Read the model definition and answer for the solid it produces. Units are mm, in the model's axes. Face numbers are marked on the shaded views. A direction names the side the tool comes from. Give positions to 0.01 mm unless a question says otherwise; leave off trailing zeros.
Autodesk Fusion 360 part; units mm, degrees
sketch "Skizze1" plane through (0, 0, 0) normal (0, 1, 0) x (1, 0, 0)
  line L0 (0, 0) -> (15, 0)
  line L1 (15, 0) -> (15, 8)
  line L2 (15, 8) -> (0, 8)
  line L3 (0, 8) -> (0, 0)
  line L4 (0, 8) -> (39.7107, 20)
  line L5 (39.7107, 20) -> (40, 19.0428)
  line L6 (40, 19.0428) -> (3.457, 8)
  line L7 (40, 19.0428) -> (40, 8)
  line L8 (40, 8) -> (15, 8)
  dimension "d1" = 15
  dimension "d2" = 8
  dimension "d3" = 1
  dimension "d4" = 20
  dimension "d5" = 40
extrude "Extrusion1" add sketch "Skizze1" along normal mid plane 50
ref_plane "Arbeitsebene1" through (39.8554, 0, -19.5214) normal (0.9572, 0, -0.2893) x (-0.2893, 0, -0.9572)
sketch "Skizze2" plane through (41.9259, 0, -12.6694) normal (0.9572, 0, -0.2893) x (-0.2893, 0, -0.9572)
  line L0 (6.658, 12.5) -> (-8.342, 12.5)
  line L1 (-8.342, 12.5) -> (-8.342, -12.5)
  line L2 (-8.342, -12.5) -> (6.658, -12.5)
  line L3 (6.658, -12.5) -> (6.658, 12.5)
  line L4 (6.658, 12.5) -> (-8.342, -12.5) construction
  line L5 (-8.342, 12.5) -> (6.658, -12.5) construction
  line L6 (6.658, -25) -> (6.658, 25)
  point P0 (-0.842, 0)
  dimension "d11" = 15
  dimension "d23" = 25
extrude "Extrusion2" cut sketch "Skizze2" against normal blind 50
sketch "Skizze3" plane through (40, 0, 0) normal (1, 0, 0) x (0, 0, -1)
  line L0 (8, 12.5) -> (19.0428, 12.5)
  line L1 (19.0428, 12.5) -> (19.0428, 25)
  line L2 (19.0428, 25) -> (8, 25)
  line L3 (8, 25) -> (8, 12.5)
  line L4 (20, -25) -> (20, 25)
  line L5 (20, 25) -> (19.0428, 25)
  line L6 (19.0428, 25) -> (19.0428, 12.5)
  line L7 (19.0428, 12.5) -> (19.0428, -12.5)
  line L8 (19.0428, -12.5) -> (19.0428, -25)
  line L9 (19.0428, -25) -> (20, -25)
  line L10 (8, 12.5) -> (19.0428, 12.5)
  line L11 (19.0428, -12.5) -> (8, -12.5)
  line L12 (8, -12.5) -> (8, -25)
  line L13 (8, -25) -> (19.0428, -25)
  line L14 (19.0428, -25) -> (19.0428, -12.5)
  spline S0 degree 5 poles (20, -12.5) (20, -13.0888) (19.7652, -14.2211) (18.7091, -15.7836) (16.1706, -17.6488) (12.3294, -19.8512) (9.7909, -21.7164) (8.7348, -23.2789) (8.5, -24.4112) (8.5, -25) knots 0 0 0 0 0 0 0.2 0.4 0.6 0.8 1 1 1 1 1 1
  line L15 (20, -11.5) -> (20, -13.5)
  line L16 (8.5, -24) -> (8.5, -26)
  dimension "d14" = 2
  dimension "d15" = 2
  dimension "d16" = 0.5
extrude "Extrusion3" cut sketch "Skizze3" against normal blind 50 contours L4 L8 L9 L14 S0 L15 | L8 L13 L14 S0
extrude "Extrusion4" add 2 faces at (31.6667, -16.6667, -8) (31.6667, 16.6667, -8) along direction (0, 0, 1) blind 0.5
mirror "Spiegeln1" about plane through (0, 0, 0) normal (0, 1, 0) of "Extrusion3"
fillet "Abrundung1" radius 2 2 edges at (20, -12.5, -12.999) (20, 12.5, -12.999)
sketch "Skizze4" plane through (0, 12.5, 0) normal (0, -1, 0) x (1, 0, 0)
  line L0 (0, -4.866) -> (40, -16.9534)
  line L1 (40, -16.9534) -> (40, -7.5)
  line L2 (40, -7.5) -> (15, -7.5)
  line L3 (15, -7.5) -> (15, 0)
  line L4 (15, 0) -> (0, 0)
  line L5 (0, 0) -> (0, -4.866)
  line L6 (15, 0) -> (40, -7.5)
extrude "Extrusion5" add sketch "Skizze4" against normal blind 0.6 contours L2 L3 L6
mirror "Spiegeln2" about plane through (0, 0, 0) normal (0, 1, 0) of "Extrusion5"
equation "d15 = d14"
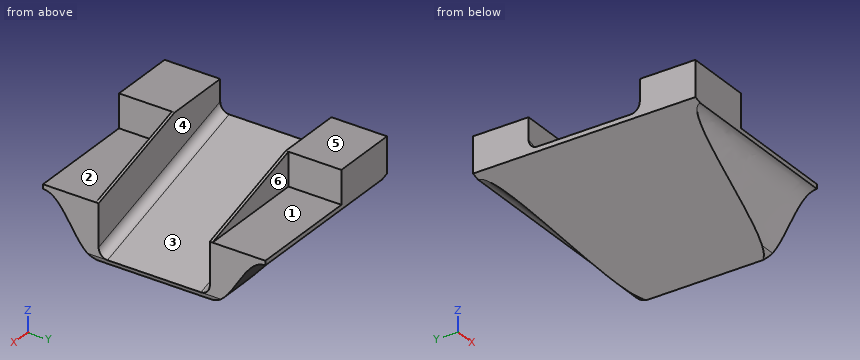
Item 1: Which of the six approach directions +Z, -Z, +X, -X, +Y, -Y give full straight-line access (tool end or side, diameter ignored) to the marked faces 1, 2 and 3?
Result set:
face 1: +Z, +X, +Y
face 2: +Z, +X, -Y
face 3: +Z, +X
Item 2: Find the intervals of material crossed by line 1 along Y through (x, z) = (23, -6); line 2 along Y through (x, z) = (2, -2); line 3 along X through (y, z) = (-13.5, -6), in increasing order.
Result set:
line 1: y = -13.1 to -12.5, 12.5 to 13.1
line 2: y = -25 to -12.5, 12.5 to 25
line 3: x = 0 to 15
Item 3: Determine the mould class of the marked faces 4, 5 and 6 for opening direction Y: pulls with the +Y half, pulls with the -Y half, needs draft (parallel to the pull), parting line crosses it, or undercut.
Result set:
face 4: undercut
face 5: needs draft
face 6: pulls with the +Y half
Item 4: Each of these flat-tipped pins is pushed along its axis until it touches: pin 1 Ø2 at (y, z) = (18, -3) entering from +X; pin 2 Ø2 at (x, z) = (25, -4) entering from +Y; pin 3 Ø6 at (x, y) = (33, -19) entering from +Z. Where does it stop, or does it pass through?
Result set:
pin 1: stops at x = 15
pin 2: stops at y = 13.1
pin 3: stops at z = -7.5
